Geometry: see drawing. Coordinates: mm, zero at the bounding-box minimum. Round coordinates to 2 decimals unless told otherwise and drop trailing zeros. Loops run counter-clockwise (first coordinate to the right, second up) from the corner with the lowest first, then second, coordinate; pieces in that order, holes last. Notation, with made-up numbers: (46.25, -32) - (85.25, -32) arc R29 ccw to (85.25, 3) - close; hole circle Ø7 at (-33.75, -8.75). An arc over 180 degrees is marked (long way). Return JSON: item names as keys, results as strings. Group by question number.
1. Material intervals for probe 1 along X at (y, z) = (5.25, 11.25); probe 2 along Z at (x, y) = (7, 0.55); probe 3 along X at (y, z) = (3.65, 6) (1 decimal), sorted ascending.
2. Section D-D on z = 1.75. Return loops of the section in (x, y) (1 decimal), and give its area (3 significant figures).
3. First-contact query: pin 1 Ø2 at (y, z) = (5, 11.5) entering from +X; pin 2 Ø2.5 at (x, z) = (128.59, 5.23) entering from +Y; pin 3 Ø8.5 at (x, z) = (130, 15.5) entering from -Y; pin 4 Ø3 at (y, z) = (3, 14) entering from -X. Flat tips, straight axial feed; report the tip coordinate or a pass-through.
4. Section C-C on x = 71.5. Return loops of the section in (y, z).
5. Section A-A on z = 12.5. Return loops of the section in (x, y).
6. Section B-B on y = 3.15. Return loops of the section in (x, z), and give its area (3 significant figures).
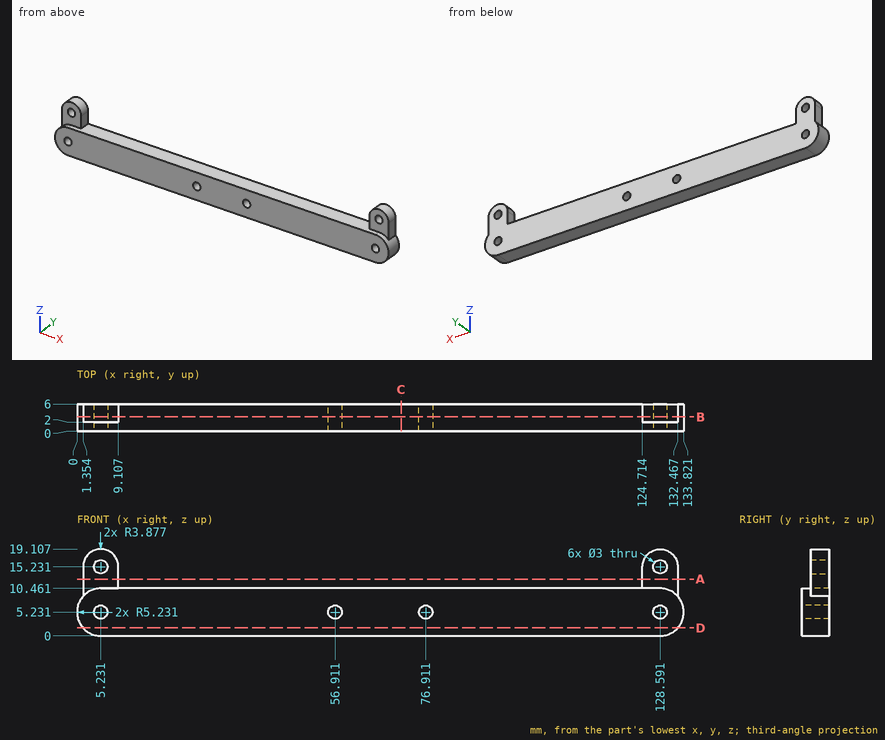
Taken from the geometry:
{
 "1": {"probe 1": "1.35 to 9.11, 124.71 to 132.47", "probe 2": "0 to 10.46", "probe 3": "0.1 to 3.9, 6.5 to 55.6, 58.2 to 75.6, 78.2 to 127.3, 129.9 to 133.8"},
 "2": {"outline": "(1.3, 0) - (132.5, 0) - (132.5, 6) - (1.3, 6) - close", "area": "787 mm2"},
 "3": {"pin 1": "x = 132.47", "pin 2": "through", "pin 3": "y = 2", "pin 4": "x = 1.35"},
 "4": {"outline": "(0, 0) - (6, 0) - (6, 10.46) - (0, 10.46) - close"},
 "5": {"outline": "(1.35, 2) - (9.11, 2) - (9.11, 6) - (1.35, 6) - close; (124.71, 2) - (132.47, 2) - (132.47, 6) - (124.71, 6) - close"},
 "6": {"outline": "(1.35, 8.74) arc R5.23 ccw to (5.23, 0) - (128.59, 0) arc R5.23 ccw to (132.47, 8.74) - (132.47, 15.23) arc R3.88 ccw to (124.71, 15.23) - (124.71, 10.46) - (9.11, 10.46) - (9.11, 15.23) arc R3.88 ccw to (1.35, 15.23) - close; hole circle Ø3 at (5.23, 5.23); hole circle Ø3 at (5.23, 15.23); hole circle Ø3 at (56.91, 5.23); hole circle Ø3 at (76.91, 5.23); hole circle Ø3 at (128.59, 5.23); hole circle Ø3 at (128.59, 15.23)", "area": "1,460 mm2"}
}
